Check sheet for the modelled part. Datum: model origin and axes. Units: mm. A direction names the side the tool comes from. Round coordinates to 2 decimals unless told otherwise and drop trailing zeros. Write each loop counter-clockwise with the first axis right and the second up, starting at its lowest first coordinate (ties: lowest second). Pieces come first, ordered by that corner, then holes. Notation, with made-up numbers: M 13,79 L 55,79 A13 cw 55,98 Z; hole C 77.5,76.5 d3. An arc over 180 degrees is marked long. Answer in a Markdown table with one row per item.
Autodesk Inventor part; units mm, degrees
ref_plane "YZ Plane" through (0, 0, 0) normal (1, 0, 0) x (0, 1, 0)
ref_plane "XZ Plane" through (0, 0, 0) normal (0, 1, 0) x (-1, 0, 0)
ref_plane "XY Plane" through (0, 0, 0) normal (0, 0, 1) x (1, 0, 0)
sketch "Sketch1" plane through (0, 0, 0) normal (0, 0, 1) x (1, 0, 0)
  circle A0 centre (0, 0) radius 6.7056
  dimension "d0" = 13.4112
extrude "Extrusion1" add sketch "Sketch1" along normal blind 5.08
fillet "Fillet1" radius 4.7625 1 edges at (-6.7056, 0, 5.08)
fillet "Fillet2" radius 0.3175 1 edges at (-6.7056, 0, 0)
sketch "Sketch2" plane through (0, 0, 5.08) normal (0, 0, 1) x (1, 0, 0)
  line L0 (0, -2.8575) -> (-2.4747, -1.4288)
  line L1 (-2.4747, -1.4288) -> (-2.4747, 1.4287)
  line L2 (-2.4747, 1.4287) -> (0, 2.8575)
  line L3 (0, 2.8575) -> (2.4747, 1.4287)
  line L4 (2.4747, 1.4287) -> (2.4747, -1.4288)
  line L5 (2.4747, -1.4288) -> (0, -2.8575)
  point P0 (0, 0)
  point P1 (0, 0)
  dimension "d5" = 5.715
extrude "Extrusion2" cut sketch "Sketch2" against normal blind 3.81
sketch "Sketch3" plane through (0, 0, 0) normal (1, 0, 0) x (0, 1, 0)
  line L0 (0, 0) -> (0, -18.288)
  line L1 (0, -18.288) -> (2.921, -18.288)
  line L2 (2.921, -18.288) -> (2.921, -4.318)
  line L3 (2.921, -4.318) -> (3.9497, -4.318)
  line L4 (3.9497, -4.318) -> (3.9497, 0)
  line L5 (6.3881, 0) -> (-6.3881, 0)
  dimension "d8" = 2.921
  dimension "d9" = 13.97
  dimension "d10" = 18.288
  dimension "d11" = 3.9497
revolve "Revolution1" add sketch "Sketch3" angle 360 about axis through (0, 0, 0) along (0, 0, -1)
fillet "Fillet3" radius 1.905 1 edges at (0, -3.9497, -4.318)
fillet "Fillet4" radius 0.3175 1 edges at (0, -3.9497, 0)
thread "Thread1"
chamfer "Chamfer1" distance 0.3175 angle 45 1 edges at (0, -2.921, -18.288)
properties part number "Axel-Male" material "Stainless Steel"
1. Draft check along X on faces 1 (the face through (-2, -4, 0)), 2 (the face through (2.852, -0.633, -11.049)), 3 (the face through (-1.255, 2.133, 3.187)). Enter one of: +X half, -X half, draft (parallel to the pull), parting line (faces both ways), or undercut.
Found:
| item | result |
|---|---|
| face 1 | draft |
| face 2 | parting line |
| face 3 | undercut |
2. Access from +Z, -Z, +X, -X, +Y, -Y to the whole of each face (thin tool, end or side, straight path). Record for faces 4 (the face through (0, 0, -18.288)), 5 (the face through (1.22, 2.153, 3.187)), 6 (the face through (-0.174, -3.946, -1.456)).
Found:
| item | result |
|---|---|
| face 4 | -Z, +X, -X, +Y, -Y |
| face 5 | +Z |
| face 6 | -Z |
3. Section check A-A, the plane z = -7. Record the cut outline in (x, y), and give its area (3 significant figures).
Found:
| item | result |
|---|---|
| outline | C 0,0 d5.84 |
| area | 26.8 mm2 |
4. Go/stop test with flat-tipped pins: pin 1 (5 mm diameter, centred on y = 3, z = -5.5, fed in from +X); pin 2 (1.4 mm diameter, centred on y = -0.5, z = 2.5, fed in from -X); pin 3 (1 mm diameter, centred on y = 1, z = -3.5, fed in from +X); pin 4 (5.5 mm diameter, centred on x = 0.5, y = 0.5, fed in from +Z). Record where each tip stops, or that it passes through.
Found:
| item | result |
|---|---|
| pin 1 | stops at x = 3.42 |
| pin 2 | stops at x = -6.45 |
| pin 3 | stops at x = 3.83 |
| pin 4 | stops at z = 5.05 |
5. Scan lines: L1, parallel to X at y = 0.5, z = 2.5; L2, parallel to X at y = 2.75, z = 2.25; L3, parallel to Y at x = 0.75, z = -3.5. Record each from-to range of solid material in increasing order.
Found:
| item | result |
|---|---|
| L1 | x = -6.16 to -2.47, 2.47 to 6.16 |
| L2 | x = -5.66 to -0.19, 0.19 to 5.66 |
| L3 | y = -3.66 to 3.66 |
